Work out the finished part from the listing and answer in its coordinate system (mm). A direction names the side the tool comes from. Round coordinates to 2 decimals unless told otherwise and drop trailing zeros. Order: outer loops, then holes, each group sorted by start corner. A loop starts at its lowest first (then second) coordinate and runs counter-clockwise, first axis right, second up.
from build123d import *

# Parameters (mm, degrees)
F1_DEPTH = 22.5
F2_R     = 2.5
F3_DEPTH = 5.001
F4_DEPTH = 5.001


with BuildPart() as f1:
    # F0 (on Front) → F1 (new body)
    with BuildSketch(Plane.XZ):
        with BuildLine():
            Line((-13.277779, 5), (-13.277779, 0))
            Line((-13.277779, 0), (46.722221, 0))
            Line((46.722221, 0), (46.722221, 5))
            Line((46.722221, 5), (34.222221, 5))
            Line((34.222221, 5), (34.222221, 17.5))
            Line((34.222221, 17.5), (29.222221, 17.5))
            ThreePointArc((29.222221, 17.5), (16.722221, 5), (4.222221, 17.5))
            Line((4.222221, 17.5), (-0.777779, 17.5))
            Line((-0.777779, 17.5), (-0.777779, 5))
            Line((-0.777779, 5), (-13.277779, 5))
        make_face()
    extrude(amount=F1_DEPTH)

    # F2 (on face) → F3 (cut, through all)
    with BuildSketch(Plane.XY.offset(5)):
        with Locations((40.472221, -11.25)):
            Circle(F2_R)
    extrude(amount=-F3_DEPTH, mode=Mode.SUBTRACT)

    # F2 (on face) → F4 (cut, through all)
    with BuildSketch(Plane.XY.offset(5)):
        with Locations((-6.440863, -11.255497)):
            Circle(F2_R)
    extrude(amount=-F4_DEPTH, mode=Mode.SUBTRACT)


solid = f1.part
Item 1: Find section C-C (z = 12.5). Write down the section's boundary in (x, y).
Item 2: Find the intervals of material crossed by line 1 along X through (y, z) = (-11.5, 2); line 2 along X through (y, z) = (-15.25, 13); line 3 along Z through (x, y) = (38, -14), in increasing order.
Item 3: Find section B-B (y = -6.5). Write down the section's boundary in (x, z), plus the area to 3 significant figures.
Item 4: Find section D-D (z = 3.5). Write down the section's boundary in (x, y), plus the area to 3 significant figures.
Item 5: Given pin 1 (1 mm diameter, centred on x = 11.5, z = 8.5, fed in from -Y); pin 2 (12 mm diameter, centred on x = 20, y = -6.5, fed in from +Z); pin 3 (8 mm diameter, centred on y = -20, z = 7, fed in from -X); pin 4 (6 mm diameter, centred on x = 39.5, y = -9, fed in from +Z), each flat-ended and moving along its own axis, determine where each tip first touches the part or whether it passes through.
Item 6: Find section A-A (x = 39). Write down the section's boundary in (y, z), plus the area to 3 significant figures.
Item 7: For a pull along X with two mould halves and no side action, classify faces 4 (the face through (46.722, -11, 2)), 5 (the face through (-0.778, -11, 11)), 6 (the face through (16.997, -11.092, 5.003)) as released by +X, released by -X, zero draft, split by the parting line, or undercut.
Item 8: A tool of negligible diameter and unlimited length cuts with its end or side. For faces 1 (the face through (16, 0, 3)), 2 (the face through (-6.9, -8.6, 5)), 3 (the face through (34.222, -11, 11)), from which of +Z, -Z, +X, -X, +Y, -Y can it reach the whole face along a straight path? Write none if from no direction.
Model answer:
1. outline: (-0.78, -22.5) - (5.27, -22.5) - (5.27, 0) - (-0.78, 0) - close; (28.18, -22.5) - (34.22, -22.5) - (34.22, 0) - (28.18, 0) - close
2. line 1: x = -13.28 to -8.93, -3.95 to 37.98, 42.96 to 46.72
2. line 2: x = -0.78 to 5.06, 28.38 to 34.22
2. line 3: z = 0 to 5
3. outline: (-13.28, 0) - (46.72, 0) - (46.72, 5) - (34.22, 5) - (34.22, 17.5) - (29.22, 17.5) arc R12.5 cw to (4.22, 17.5) - (-0.78, 17.5) - (-0.78, 5) - (-13.28, 5) - close
3. area: 492 mm2
4. outline: (-13.28, -22.5) - (46.72, -22.5) - (46.72, 0) - (-13.28, 0) - close; hole circle Ø5 at (-6.44, -11.26); hole circle Ø5 at (40.47, -11.25)
4. area: 1,310 mm2
5. pin 1: passes through
5. pin 2: stops at z = 9.12
5. pin 3: stops at x = -13.28
5. pin 4: stops at z = 5
6. outline: (-22.5, 0) - (-13.27, 0) - (-13.27, 5) - (-22.5, 5) - close; (-9.23, 0) - (0, 0) - (0, 5) - (-9.23, 5) - close
6. area: 92.3 mm2
7. face 4: released by +X
7. face 5: released by -X
7. face 6: undercut
8. face 1: +Z, -Z, +X, -X, +Y
8. face 2: +Z, -X, +Y, -Y
8. face 3: +Z, +X, +Y, -Y
